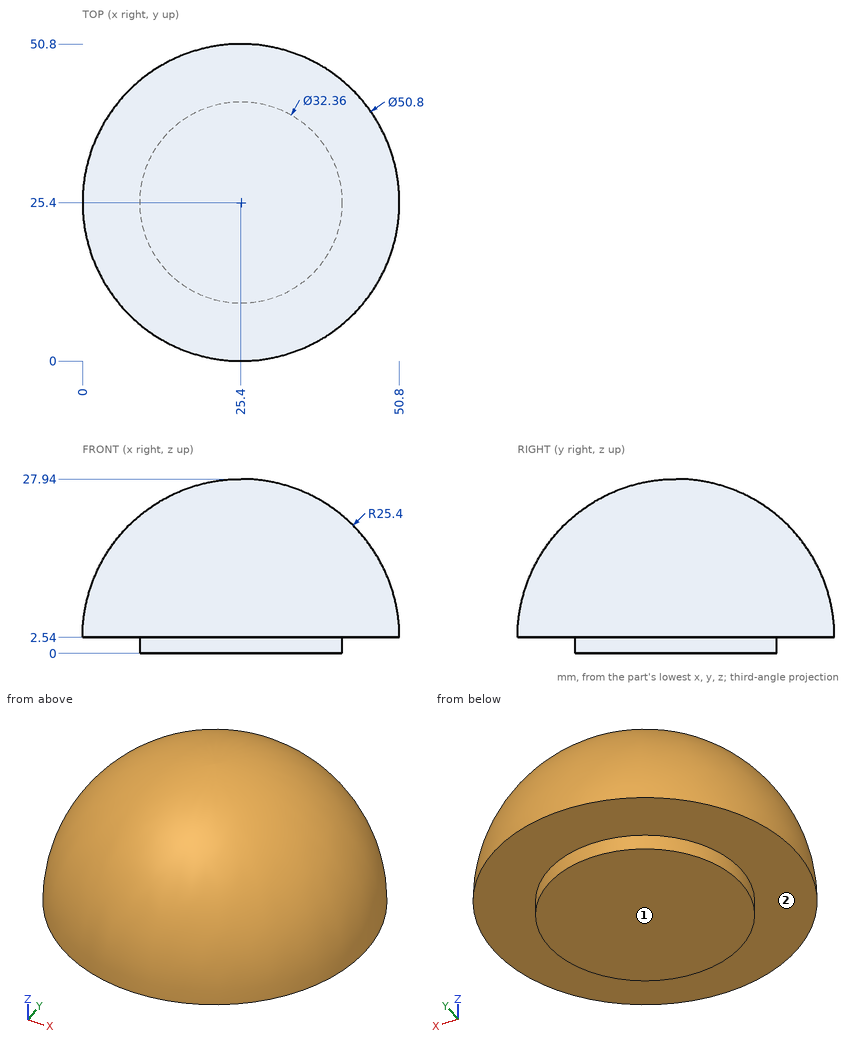
Check sheet for the drawn part. Datum: minimum x, y, z corner. Units: mm. A direction names the side the tool comes from. Round coordinates to 2 decimals unless told otherwise and drop trailing zeros. Put each result on its own line as item: value.
(1) Go/stop test with flat-tipped pins: pin 1 Ø1 at (x, z) = (15.5, 16.5) entering from +Y; pin 2 Ø12 at (x, y) = (10.5, 31.5) entering from +Z (1 decimal); pin 3 Ø8 at (y, z) = (14.5, 18) entering from +X. Record where each tip stops, or that it passes through.
Values found:
pin 1: stops at y = 44.61
pin 2: stops at z = 25.8
pin 3: stops at x = 45.96
(2) Material ranges on line 1 (Y direction, x = 26, z = 2.75); line 2 (Z direction, x = 23, y = 18), recorded low to high.
Values found:
line 1: y = 0.01 to 50.79
line 2: z = 0 to 26.72
(3) Tool access check on the marked faces 1 and 2. Record the directions out of +Z, -Z, +X, -X, +Y, -Y that give a thin tool (end or side, any length) a straight path to the whole face; none if there is none.
Values found:
face 1: -Z, +X, -X, +Y, -Y
face 2: -Z
